Input: part model. Units: mm. Frame: model coordinates. Coordinates: 2 decimals unless noted, no trailing zeros. Order: outer loops, then holes, each group sorted by start corner. A loop starts at its lowest first (then second) coordinate and runs counter-clockwise, first axis right, second up. Notation, with made-up numbers: (57, 23.5) - (102, 23.5) arc R37 cw to (102, 62.5) - close; hole circle Ø1 at (-34, -26.75). An arc over 180 degrees is marked (long way). One line per question, with ' | ' between items. Start each with the question number.
```python
from build123d import *

# Parameters (mm, degrees)
BOSS_EXTRU_1_DEPTH       = 15
CONG_10_R                = 10
ENL_V_MAT_EXTRU_13_REACH = 393.106
ESQUISSE13_W             = 20
ESQUISSE13_H             = 143.033455182
ESQUISSE13_H_2           = 181.308681646
CONG_12_R                = 10
ENL_V_MAT_EXTRU_14_REACH = 377.805
ESQUISSE14_R             = 1.6


with BuildPart() as part:
    # Esquisse1 → Boss.-Extru.1 (new body)
    with BuildSketch(Plane(origin=(0, 0, 0), x_dir=(1, 0, 0), z_dir=(0, 1, 0))):
        Polygon((-76.643189126, -51.401333399), (63.356810874, 43.598666601), (163.356810874, 43.598666601), (303.356810874, -51.401333399), (303.356810874, -151.401333399), (163.356810874, -246.401333399), (63.356810874, -246.401333399), (-76.643189126, -151.401333399), align=None)
    extrude(amount=BOSS_EXTRU_1_DEPTH)

    # Congé10
    cong_10_edges = [part.edges().sort_by_distance(p)[0] for p in [
        (-76.643189126, 7.5, 51.401333399),
        (63.356810874, 7.5, -43.598666601),
        (163.356810874, 7.5, -43.598666601),
        (303.356810874, 7.5, 51.401333399),
        (303.356810874, 7.5, 151.401333399),
        (163.356810874, 7.5, 246.401333399),
        (63.356810874, 7.5, 246.401333399),
        (-76.643189126, 7.5, 151.401333399),
    ]]
    fillet(cong_10_edges, radius=CONG_10_R)

    # Esquisse13 → Enlèv. mat.-Extru.13 (cut, up to next)
    with BuildSketch(Plane(origin=(0, 15, 0), x_dir=(1, 0, 0), z_dir=(0, 1, 0)), mode=Mode.PRIVATE) as enl_v_mat_extru_13_sk1:
        with Locations((-66.643189126, -101.968599131)):
            Rectangle(ESQUISSE13_W, ESQUISSE13_H)
    enl_v_mat_extru_13_tool1 = extrude(enl_v_mat_extru_13_sk1.sketch, amount=-ENL_V_MAT_EXTRU_13_REACH, mode=Mode.PRIVATE) & part.part
    # Esquisse13 → Enlèv. mat.-Extru.13 (cut, up to next)
    with BuildSketch(Plane(origin=(0, 15, 0), x_dir=(1, 0, 0), z_dir=(0, 1, 0)), mode=Mode.PRIVATE) as enl_v_mat_extru_13_sk2:
        with Locations((293.356810874, -101.059068944)):
            Rectangle(ESQUISSE13_W, ESQUISSE13_H_2)
    enl_v_mat_extru_13_tool2 = extrude(enl_v_mat_extru_13_sk2.sketch, amount=-ENL_V_MAT_EXTRU_13_REACH, mode=Mode.PRIVATE) & part.part
    add(enl_v_mat_extru_13_tool1.solids().sort_by_distance((-66.643189, 15, 101.968599))[0], mode=Mode.SUBTRACT)
    add(enl_v_mat_extru_13_tool2.solids().sort_by_distance((293.356811, 15, 101.059069))[0], mode=Mode.SUBTRACT)

    # Congé12
    cong_12_edges = [part.edges().sort_by_distance(p)[0] for p in [
        (-56.643189126, 7.5, 37.829904828),
        (-56.643189126, 7.5, 164.97276197),
        (283.356810874, 7.5, 37.829904828),
        (283.356810874, 7.5, 164.97276197),
    ]]
    fillet(cong_12_edges, radius=CONG_12_R)

    # Esquisse14 → Enlèv. mat.-Extru.14 (cut, up to next)
    with BuildSketch(Plane(origin=(0, 15, 0), x_dir=(1, 0, 0), z_dir=(0, 1, 0)), mode=Mode.PRIVATE) as enl_v_mat_extru_14_sk1:
        with Locations(Location((-42.643189126, -51.403530316, 0), (0, 0, 270))):
            Circle(ESQUISSE14_R)
    enl_v_mat_extru_14_tool1 = extrude(enl_v_mat_extru_14_sk1.sketch, amount=-ENL_V_MAT_EXTRU_14_REACH, mode=Mode.PRIVATE) & part.part
    # Esquisse14 → Enlèv. mat.-Extru.14 (cut, up to next)
    with BuildSketch(Plane(origin=(0, 15, 0), x_dir=(1, 0, 0), z_dir=(0, 1, 0)), mode=Mode.PRIVATE) as enl_v_mat_extru_14_sk2:
        with Locations(Location((-42.643189126, -151.403530316, 0), (0, 0, 270))):
            Circle(ESQUISSE14_R)
    enl_v_mat_extru_14_tool2 = extrude(enl_v_mat_extru_14_sk2.sketch, amount=-ENL_V_MAT_EXTRU_14_REACH, mode=Mode.PRIVATE) & part.part
    # Esquisse14 → Enlèv. mat.-Extru.14 (cut, up to next)
    with BuildSketch(Plane(origin=(0, 15, 0), x_dir=(1, 0, 0), z_dir=(0, 1, 0)), mode=Mode.PRIVATE) as enl_v_mat_extru_14_sk3:
        with Locations(Location((73.359258963, 29.598666601, 0), (0, 0, 270))):
            Circle(ESQUISSE14_R)
    enl_v_mat_extru_14_tool3 = extrude(enl_v_mat_extru_14_sk3.sketch, amount=-ENL_V_MAT_EXTRU_14_REACH, mode=Mode.PRIVATE) & part.part
    # Esquisse14 → Enlèv. mat.-Extru.14 (cut, up to next)
    with BuildSketch(Plane(origin=(0, 15, 0), x_dir=(1, 0, 0), z_dir=(0, 1, 0)), mode=Mode.PRIVATE) as enl_v_mat_extru_14_sk4:
        with Locations(Location((153.359258963, 29.598666601, 0), (0, 0, 270))):
            Circle(ESQUISSE14_R)
    enl_v_mat_extru_14_tool4 = extrude(enl_v_mat_extru_14_sk4.sketch, amount=-ENL_V_MAT_EXTRU_14_REACH, mode=Mode.PRIVATE) & part.part
    # Esquisse14 → Enlèv. mat.-Extru.14 (cut, up to next)
    with BuildSketch(Plane(origin=(0, 15, 0), x_dir=(1, 0, 0), z_dir=(0, 1, 0)), mode=Mode.PRIVATE) as enl_v_mat_extru_14_sk5:
        with Locations(Location((269.356810874, -51.399136482, 0), (0, 0, 270))):
            Circle(ESQUISSE14_R)
    enl_v_mat_extru_14_tool5 = extrude(enl_v_mat_extru_14_sk5.sketch, amount=-ENL_V_MAT_EXTRU_14_REACH, mode=Mode.PRIVATE) & part.part
    # Esquisse14 → Enlèv. mat.-Extru.14 (cut, up to next)
    with BuildSketch(Plane(origin=(0, 15, 0), x_dir=(1, 0, 0), z_dir=(0, 1, 0)), mode=Mode.PRIVATE) as enl_v_mat_extru_14_sk6:
        with Locations(Location((269.356810874, -141.399136482, 0), (0, 0, 270))):
            Circle(ESQUISSE14_R)
    enl_v_mat_extru_14_tool6 = extrude(enl_v_mat_extru_14_sk6.sketch, amount=-ENL_V_MAT_EXTRU_14_REACH, mode=Mode.PRIVATE) & part.part
    add(enl_v_mat_extru_14_tool1.solids().sort_by_distance((-42.643189, 15, 51.40353))[0], mode=Mode.SUBTRACT)
    add(enl_v_mat_extru_14_tool2.solids().sort_by_distance((-42.643189, 15, 151.40353))[0], mode=Mode.SUBTRACT)
    add(enl_v_mat_extru_14_tool3.solids().sort_by_distance((73.359259, 15, -29.598667))[0], mode=Mode.SUBTRACT)
    add(enl_v_mat_extru_14_tool4.solids().sort_by_distance((153.359259, 15, -29.598667))[0], mode=Mode.SUBTRACT)
    add(enl_v_mat_extru_14_tool5.solids().sort_by_distance((269.356811, 15, 51.399136))[0], mode=Mode.SUBTRACT)
    add(enl_v_mat_extru_14_tool6.solids().sort_by_distance((269.356811, 15, 141.399136))[0], mode=Mode.SUBTRACT)


solid = part.part
```
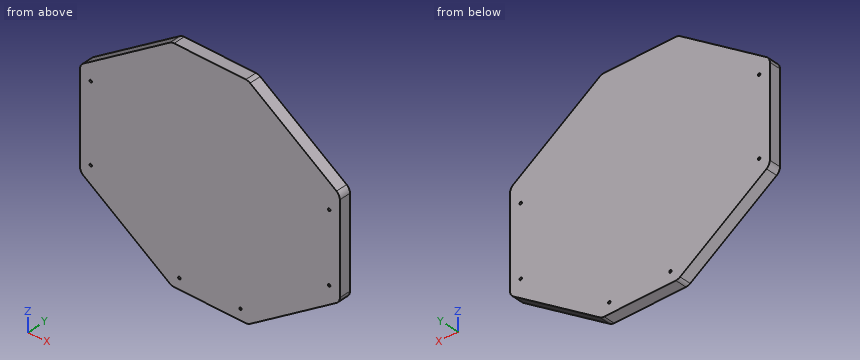
(1) Section C-C (x = 199.5). Output: boundary loops of the cut face in (y, z).
(2) Pin query (flat end, axial travel): pin 1 (4 mm diameter, centred on y = 11, z = 199.5, fed in from -X); pin 2 (4 mm diameter, centred on x = 21, y = 7.5, fed in from -Z); pin 3 (1.5 mm diameter, centred on y = 4, z = 189.5, fed in from -X). Return the tip coordinate at first contact, or that it passes through.
(3) Section A-A (y = 12). Output: boundary loops of the cut face in (x, z).
(4) Material intervals for line 1 along X through (y, z) = (13, 160.5); line 2 along Z through (x, y) = (4.5, 2.25); line 3 along X through (y, z) = (3.25, -6.5), sorted ascending. Write a range as from..to.
(5) Section B-B (z = 27). Output: boundary loops of the cut face in (x, y), then the cut area to 3 significant figures.
Worked answers:
1) outline: (0, -19.07) - (15, -19.07) - (15, 221.88) - (0, 221.88) - close
2) pin 1: stops at x = -8.71 | pin 2: stops at z = -16.21 | pin 3: stops at x = -21.6
3) outline: (-56.64, 43.13) arc R10 ccw to (-52.26, 34.85) - (60.81, -41.87) arc R10 ccw to (66.43, -43.6) - (160.28, -43.6) arc R10 ccw to (165.9, -41.87) - (278.97, 34.85) arc R10 ccw to (283.36, 43.13) - (283.36, 159.67) arc R10 ccw to (278.97, 167.95) - (165.9, 244.68) arc R10 ccw to (160.28, 246.4) - (66.43, 246.4) arc R10 ccw to (60.81, 244.68) - (-52.26, 167.95) arc R10 ccw to (-56.64, 159.67) - close; hole circle Ø3.2 at (-42.64, 51.4); hole circle Ø3.2 at (-42.64, 151.4); hole circle Ø3.2 at (73.36, -29.6); hole circle Ø3.2 at (153.36, -29.6); hole circle Ø3.2 at (269.36, 51.4); hole circle Ø3.2 at (269.36, 141.4)
4) line 1: x = -56.61..283.32 | line 2: z = -3.66..206.46 | line 3: x = 8.69..218.03
5) outline: (-40.68, 0) - (267.4, 0) - (267.4, 15) - (-40.68, 15) - close | area: 4,620 mm²
